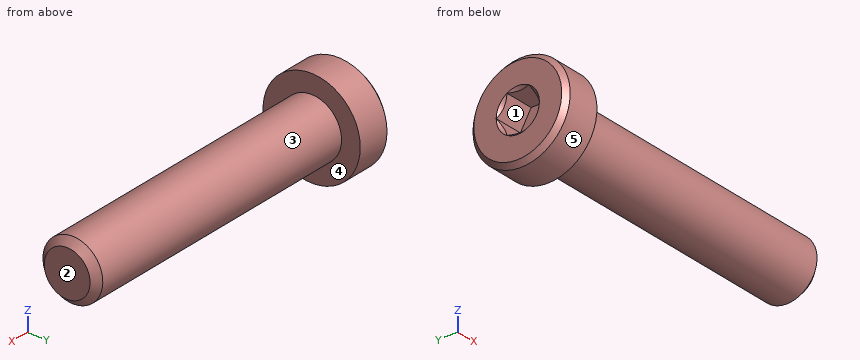
from build123d import *

# Parameters (mm, degrees)
SKETCH2_R           = 4
BOSS_EXTRUDE1_DEPTH = 22
CHAMFER1_SIZE       = 0.9375
CUT_EXTRUDE1_DEPTH  = 3.95


with BuildPart() as part:
    # Sketch2 → Boss-Extrude1 (new body)
    with BuildSketch(Plane(origin=(20, 0, 0), x_dir=(0, 0, -1), z_dir=(1, 0, 0))):
        Circle(SKETCH2_R)
    extrude(amount=-BOSS_EXTRUDE1_DEPTH)

    # Chamfer1
    chamfer1_edges = [part.edges().sort_by_distance(p)[0] for p in [
        (20, 0, 4),
    ]]
    chamfer(chamfer1_edges, length=CHAMFER1_SIZE)

    # Sketch10 → Revolve2 (revolve)
    with BuildSketch(Plane.XY, mode=Mode.PRIVATE) as revolve2_sk:
        Polygon((0.309401077, 0), (-2, 4), (-20, 4), (-20, 0), align=None)
    revolve(revolve2_sk.sketch.rotate(Axis((-20, 0, 0), (1, 0, 0)), 270), axis=Axis((-20, 0, 0), (1, 0, 0)))

    # Sketch6 → Revolve1 (revolve)
    with BuildSketch(Plane.XY):
        Polygon((-24.375, 6.5), (-25, 5.875), (-25, 0), (-20, 0), (-20, 6.5), align=None)
    revolve(axis=Axis((-20, 0, 0), (-1, 0, 0)))

    # Sketch4 → Cut-Extrude1 (cut)
    with BuildSketch(Plane(origin=(-25, 0, 0), x_dir=(0, 0, -1), z_dir=(1, 0, 0))):
        Polygon((0, 2.886751346), (-2.5, 1.443375673), (-2.5, -1.443375673), (0, -2.886751346), (2.5, -1.443375673), (2.5, 1.443375673), align=None)
    extrude(amount=CUT_EXTRUDE1_DEPTH, mode=Mode.SUBTRACT)

    # Cut-Extrude2 cone 1 section (through the dimple's axis) → Cut-Extrude2 (revolve, cut)
    with BuildSketch(Plane(origin=(-25, 0, 0), x_dir=(0, 0, 1), z_dir=(0, 1, 0))):
        Polygon((0, 0), (2.886751346, 0), (0, 2.886751346), align=None)
    revolve(axis=Axis((-25, 0, 0), (1, 0, 0)), mode=Mode.SUBTRACT)


solid = part.part
Geometry: final body of the model. Coordinates: model frame, mm. Face numbers are marked on the shaded views. A direction names the side the tool comes from. Give positions to 0.01 mm unless a question says otherwise; leave off trailing zeros. Order: outer loops, then holes, each group sorted by start corner. A loop starts at its lowest first (then second) coordinate and runs counter-clockwise, first axis right, second up. Notation, with made-up numbers: (-8, 39) -> (14, 39) arc R19 cw to (14, 52) -> close; hole circle Ø2 at (1.5, 44.25). An arc over 180 degrees is marked (long way). Write each question's results on one line, items separated by ' | '.
1) First-contact query: pin 1 Ø6 at (y, z) = (3.5, 5) entering from -X; pin 2 Ø1.5 at (x, y) = (8.5, -5) entering from +Z; pin 3 Ø1.5 at (y, z) = (1.5, 0) entering from -X; pin 4 Ø3 at (x, y) = (-11, 0) entering from +Z. Flat tips, straight axial feed; report the tip coordinate or a pass-through.
Geometry says:
pin 1: stops at x = -25 | pin 2: passes through | pin 3: stops at x = -21.05 | pin 4: stops at z = 4
2) Set-up query: the marked faces 4 and 5. Return all of +Z, -Z, +X, -X, +Y, -Y with unobstructed straight access to the full face (end or side cutting, diameter ignored); none if empty.
Geometry says:
face 4: +X | face 5: +X, -X
3) Cut plane B-B (x = 4). Output: boundary loops of the cut face in (y, z).
Geometry says:
outline: circle Ø8 at (0, 0)
4) Draft query along Y for the marked faces 1, 2 and 3. Return one class per face: released by +Y, released by -Y, zero draft, split by the parting line, or undercut.
Geometry says:
face 1: undercut | face 2: zero draft | face 3: split by the parting line
5) Line query: line 1 along X through (y, z) = (0, -1.25); line 2 along X through (y, z) = (3.5, -2.5); line 3 along Y through (x, z) = (14, 1). Output: solid intervals per line, ascending.
Geometry says:
line 1: x = -21.05 to 20 | line 2: x = -25 to -20 | line 3: y = -3.87 to 3.87
6) Cut plane C-C (x = -20.5). Output: boundary loops of the cut face in (y, z), and give its area (3 significant figures).
Geometry says:
outline: circle Ø13 at (0, 0) | area: 133 mm²
